Read the model definition and answer for the solid it produces. Units are mm, in the model's axes. A direction names the side the tool comes from. Coordinates: 2 decimals unless noted, no trailing zeros. Loops run counter-clockwise (first coordinate to the right, second up) from the corner with the lowest first, then second, coordinate; pieces in that order, holes last. Notation, with made-up numbers: (-37.5, 40.25) -> (-24.5, 40.25) arc R21 cw to (-24.5, 72.25) -> close; hole circle Ø5 at (83.25, -36). An arc over 180 degrees is marked (long way). Answer as a JSON object with one key per item and string values. Group by question number.
1) Consider probe 1 along Y at (x, z) = (14.5, 5); probe 2 along Z at (x, y) = (-10, 6.5); probe 3 along Z at (x, y) = (-12, -32). Determine where each line is inside the solid, lowest interval first. Write a range as [from, to].
2) Section D-D, the plane y = 25.5 is taken. Give the vertices of the cut face in (x, z), plus the area to 3 significant figures.
3) Which of the six approach directions +Z, -Z, +X, -X, +Y, -Y give full straight-line access (tool end or side, diameter ignored) to faces 5 (the face through (21.038, -42, -15)), 6 (the face through (-2, -60, -14.55)), 7 (the face through (17.738, -41.093, -15.426)), 8 (the face through (-2, -25.939, -15))?
4) Section C-C, the plane z = 15.5 is taken. Give the vertices of the cut face in (x, y).
5) Determine the mould class of faces 1 (the face through (-2, -42, -13.55)), 2 (the face through (34.338, -11, 8)), 3 (the face through (2, -52, -1.64)), 4 (the face through (-2, -42, -17.25)) for opening direction Z: released by +Z, released by -Z, zero draft, split by the parting line, or undercut.
6) Flat-ended cylindrical pins translate along their axes: P1, Ø3.5, axis at x = 30.84, y = -52.93, coming from the -Z side; P2, Ø10, axis at x = -4.5, z = 3, coming from the -Y side; P3, Ø4, axis at y = -40, z = -15.5, coming from the -X side; P4, Ø1.5, axis at y = 22.5, z = -0.5, coming from the +X side. Find the tip coordinate at first contact, or state that the pin passes through.
7) Section A-A, the plane y = -31 is taken. Give the vertices of the cut face in (x, z), plus the area to 3 significant figures.
8) Section B-B, the plane x = -9 is taken. Give the vertices of the cut face in (y, z).
from build123d import *

# Parameters (mm, degrees)
SKETCH1_W            = 65
SKETCH1_H            = 91.3
BOSS_EXTRUDE2_DEPTH  = 18.2
SKETCH12_W           = 65
SKETCH12_H           = 9
BOSS_EXTRUDE7_DEPTH  = 1.64
SKETCH13_W           = 34.2
SKETCH13_H           = 0.25
BOSS_EXTRUDE8_DEPTH  = 5.61
BOSS_EXTRUDE13_DEPTH = 34.2
SKETCH19_W           = 34.2
SKETCH19_H           = 0.25
BOSS_EXTRUDE14_DEPTH = 4.1
SKETCH20_W           = 45.4
SKETCH20_H           = 3.7
BOSS_EXTRUDE15_DEPTH = 32
SKETCH21_R           = 1.4
CUT_EXTRUDE2_DEPTH   = 32
SKETCH22_R           = 1.4
CUT_EXTRUDE3_DEPTH   = 61
SKETCH23_R           = 1.4
CUT_EXTRUDE4_DEPTH   = 61
SKETCH24_R           = 1.4
CUT_EXTRUDE5_DEPTH   = 61
SKETCH25_R           = 1.3
CUT_EXTRUDE6_DEPTH   = 10
SKETCH26_R           = 1.3
CUT_EXTRUDE7_DEPTH   = 10
SKETCH27_R           = 1.4
CUT_EXTRUDE9_DEPTH   = 1500


with BuildPart() as part:
    # Sketch1 → Boss-Extrude2 (new body)
    with BuildSketch(Plane.XY):
        with Locations((1.837659334, -10.779179331)):
            Rectangle(SKETCH1_W, SKETCH1_H)
    extrude(amount=BOSS_EXTRUDE2_DEPTH)

    # Sketch12 → Boss-Extrude7 (add)
    with BuildSketch(Plane(origin=(0, 0, 0), x_dir=(-1, 0, 0), z_dir=(0, 0, -1))):
        with Locations((-1.837659334, -51.929179331)):
            Rectangle(SKETCH12_W, SKETCH12_H)
    extrude(amount=BOSS_EXTRUDE7_DEPTH)

    # Sketch13 → Boss-Extrude8 (add)
    with BuildSketch(Plane.XZ.offset(56.429179331)):
        with Locations((-1.662340666, 3.075)):
            Rectangle(SKETCH13_W, SKETCH13_H)
    extrude(amount=BOSS_EXTRUDE8_DEPTH)

    # Sketch18 → Boss-Extrude13 (add)
    with BuildSketch(Plane.ZY.offset(18.762340666)):
        with BuildLine():
            Line((3.2, -62.039179331), (2.95, -62.039179331))
            ThreePointArc((2.95, -62.039179331), (-5.8, -70.789179331), (-14.55, -62.039179331))
            Line((-14.55, -62.039179331), (-14.8, -62.039179331))
            ThreePointArc((-14.8, -62.039179331), (-5.8, -71.039179331), (3.2, -62.039179331))
        make_face()
    extrude(amount=-BOSS_EXTRUDE13_DEPTH)

    # Sketch19 → Boss-Extrude14 (add)
    with BuildSketch(Plane(origin=(0, -62.039179331, 0), x_dir=(1, 0, 0), z_dir=(0, 1, 0))):
        with Locations((-1.662340666, 14.675)):
            Rectangle(SKETCH19_W, SKETCH19_H)
    extrude(amount=BOSS_EXTRUDE14_DEPTH)

    # Sketch20 → Boss-Extrude15 (add)
    with BuildSketch(Plane(origin=(0, -57.939179331, 0), x_dir=(1, 0, 0), z_dir=(0, 1, 0))):
        with Locations((-1.662340666, 15.4)):
            Rectangle(SKETCH20_W, SKETCH20_H)
    extrude(amount=BOSS_EXTRUDE15_DEPTH)

    # Sketch21 → Cut-Extrude2 (cut)
    with BuildSketch(Plane.XY.offset(18.2)):
        with Locations((30.837659334, 31.370820669)):
            Circle(SKETCH21_R)
    extrude(amount=-CUT_EXTRUDE2_DEPTH, mode=Mode.SUBTRACT)

    # Sketch22 → Cut-Extrude3 (cut)
    with BuildSketch(Plane.XY.offset(18.2)):
        with Locations((-27.162340666, 31.370820669)):
            Circle(SKETCH22_R)
    extrude(amount=-CUT_EXTRUDE3_DEPTH, mode=Mode.SUBTRACT)

    # Sketch23 → Cut-Extrude4 (cut)
    with BuildSketch(Plane.XY.offset(18.2)):
        with Locations((30.837659334, -52.929179331)):
            Circle(SKETCH23_R)
    extrude(amount=-CUT_EXTRUDE4_DEPTH, mode=Mode.SUBTRACT)

    # Sketch24 → Cut-Extrude5 (cut)
    with BuildSketch(Plane.XY.offset(18.2)):
        with Locations((-27.162340666, -52.929179331)):
            Circle(SKETCH24_R)
    extrude(amount=-CUT_EXTRUDE5_DEPTH, mode=Mode.SUBTRACT)

    # Sketch25 → Cut-Extrude6 (cut)
    with BuildSketch(Plane(origin=(0, 0, -17.25), x_dir=(-1, 0, 0), z_dir=(0, 0, -1))):
        with Locations((21.662340666, -39.939179331)):
            Circle(SKETCH25_R)
    extrude(amount=-CUT_EXTRUDE6_DEPTH, mode=Mode.SUBTRACT)

    # Sketch26 → Cut-Extrude7 (cut)
    with BuildSketch(Plane(origin=(0, 0, -17.25), x_dir=(-1, 0, 0), z_dir=(0, 0, -1))):
        with Locations((-18.337659334, -39.939179331)):
            Circle(SKETCH26_R)
    extrude(amount=-CUT_EXTRUDE7_DEPTH, mode=Mode.SUBTRACT)

    # Sketch27 → Cut-Extrude9 (cut)
    with BuildSketch(Plane.XY.offset(18.2)):
        with Locations((30.837659334, -23.429179331)):
            Circle(SKETCH27_R)
    extrude(amount=-CUT_EXTRUDE9_DEPTH, mode=Mode.SUBTRACT)


solid = part.part
Determined:
{
 "1": {"probe 1": "[-56.43, 34.87]", "probe 2": "[0, 18.2]", "probe 3": "[-17.25, -13.55], [0, 18.2]"},
 "2": {"outline": "(-30.66, 0) -> (34.34, 0) -> (34.34, 18.2) -> (-30.66, 18.2) -> close", "area": "1,180 mm²"},
 "3": {"face 5": "-Z, +X, +Y, -Y", "face 6": "+X, -X", "face 7": "-Z", "face 8": "-Z, +X, -X, +Y"},
 "4": {"outline": "(-30.66, -56.43) -> (34.34, -56.43) -> (34.34, 34.87) -> (-30.66, 34.87) -> close; hole circle Ø2.8 at (-27.16, -52.93); hole circle Ø2.8 at (-27.16, 31.37); hole circle Ø2.8 at (30.84, -52.93); hole circle Ø2.8 at (30.84, -23.43); hole circle Ø2.8 at (30.84, 31.37)"},
 "5": {"face 1": "undercut", "face 2": "zero draft", "face 3": "undercut", "face 4": "released by -Z"},
 "6": {"P1": "z = -1.64", "P2": "y = -70.2", "P3": "x = -24.36", "P4": "x = 34.34"},
 "7": {"outline": "(-30.66, 0) -> (34.34, 0) -> (34.34, 18.2) -> (-30.66, 18.2) -> close; (-24.36, -17.25) -> (21.04, -17.25) -> (21.04, -13.55) -> (-24.36, -13.55) -> close", "area": "1,350 mm²"},
 "8": {"outline": "(-62.04, -14.8) -> (-57.94, -14.8) -> (-57.94, -17.25) -> (-25.94, -17.25) -> (-25.94, -13.55) -> (-57.94, -13.55) -> (-57.94, -14.55) -> (-62.04, -14.55) arc R8.75 cw to (-62.04, 2.95) -> (-56.43, 2.95) -> (-56.43, -1.64) -> (-47.43, -1.64) -> (-47.43, 0) -> (34.87, 0) -> (34.87, 18.2) -> (-56.43, 18.2) -> (-56.43, 3.2) -> (-62.04, 3.2) arc R9 ccw to start"}
}
